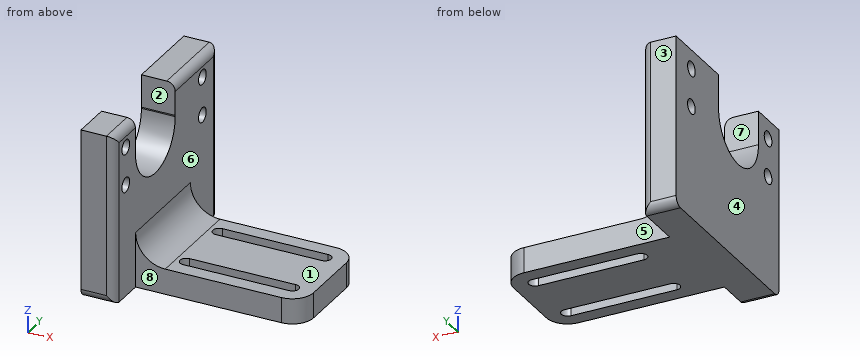
from build123d import *

# Parameters (mm, degrees)
F0_W     = 39.5
F0_H     = 25
F1_DEPTH = 6
F2_R     = 5
F3_W     = 8
F3_H     = 47
F4_DEPTH = 25
F5_R     = 7
F6_DEPTH = 40
F7_R     = 1.75
F8_DEPTH = 25
F9_R     = 2


with BuildPart() as f1:
    # F0 (on Top) → F1 (new body)
    with BuildSketch(Plane.XY):
        with Locations((19.75, -12.5)):
            Rectangle(F0_W, F0_H)
        with BuildLine():
            ThreePointArc((9.428176, -21.5), (7.928176, -20), (9.428176, -18.5))
            Line((9.428176, -18.5), (34.428176, -18.5))
            ThreePointArc((34.428176, -18.5), (36.00043, -19.963218), (34.5, -21.5))
            Line((34.5, -21.5), (9.428176, -21.5))
        make_face(mode=Mode.SUBTRACT)
        with BuildLine():
            ThreePointArc((9.428176, -6.5), (7.928176, -5), (9.428176, -3.5))
            Line((9.428176, -3.5), (34.428176, -3.5))
            ThreePointArc((34.428176, -3.5), (35.928176, -5), (34.428176, -6.5))
            Line((34.428176, -6.5), (9.428176, -6.5))
        make_face(mode=Mode.SUBTRACT)
    extrude(amount=F1_DEPTH)

    # F2
    f2_edges = [f1.edges().sort_by_distance(p)[0] for p in [
        (39.5, 0, 3),
        (39.5, -25, 3),
    ]]
    fillet(f2_edges, radius=F2_R)

    # F3 (on Top) → F4 (join)
    with BuildSketch(Plane.XY):
        with Locations((-4, -11)):
            Rectangle(F3_W, F3_H)
    extrude(amount=F4_DEPTH)

    # F5
    f5_edges = [f1.edges().sort_by_distance(p)[0] for p in [
        (0, -12.5, 6),
        (0, -34.5, 12.5),
        (0, 12.5, 12.5),
    ]]
    fillet(f5_edges, radius=F5_R)

    # F3 (on Top) → F6 (join)
    with BuildSketch(Plane.XY):
        with Locations((-4, -11)):
            Rectangle(F3_W, F3_H)
    extrude(amount=F6_DEPTH)

    # F7 (on Right) → F8 (cut)
    with BuildSketch(Plane.YZ):
        with Locations((-29.5, 35.5)):
            Circle(F7_R)
        with Locations((5.5, 35.5)):
            Circle(F7_R)
        with Locations((5.5, 26.5)):
            Circle(F7_R)
        with Locations((-29.5, 26.5)):
            Circle(F7_R)
        with BuildLine():
            ThreePointArc((-25.098021, 32), (-16, 22.901979), (-6.901979, 32))
            ThreePointArc((-6.901979, 32), (-6.903109, 32.143378), (-6.906498, 32.286721))
            ThreePointArc((-6.906498, 32.286721), (-8.276915, 36.809152), (-11.730835, 40.03419))
            Line((-11.730835, 40.03419), (-20.269165, 40.03419))
            ThreePointArc((-20.269165, 40.03419), (-23.797914, 36.686845), (-25.098021, 32))
        make_face()
        with BuildLine():
            ThreePointArc((-11.730835, 40.03419), (-8.276915, 36.809152), (-6.906498, 32.286721))
            Line((-6.906498, 32.286721), (-6.906498, 40.03419))
            Line((-6.906498, 40.03419), (-11.730835, 40.03419))
        make_face()
        with BuildLine():
            Line((-25.098021, 40.03419), (-25.098021, 32))
            ThreePointArc((-25.098021, 32), (-23.797914, 36.686845), (-20.269165, 40.03419))
            Line((-20.269165, 40.03419), (-25.098021, 40.03419))
        make_face()
        with BuildLine():
            Line((-20.269165, 40.03419), (-11.730835, 40.03419))
            ThreePointArc((-11.730835, 40.03419), (-16, 41.098021), (-20.269165, 40.03419))
        make_face()
    extrude(amount=-F8_DEPTH, mode=Mode.SUBTRACT)

    # F9
    f9_edges = [f1.edges().sort_by_distance(p)[0] for p in [
        (0, 2.796751, 40),
        (0, -29.79901, 40),
        (0, -34.5, 20),
        (0, 12.5, 20),
        (-4, 12.5, 0),
        (-4, -34.5, 0),
    ]]
    fillet(f9_edges, radius=F9_R)


solid = f1.part
Read the model definition and answer for the solid it produces. Units are mm, in the model's axes. Face numbers are marked on the shaded views. A direction names the side the tool comes from. Give positions to 0.01 mm unless a question says otherwise; leave off trailing zeros. Loops run counter-clockwise (first coordinate to the right, second up) from the corner with the lowest first, then second, coordinate; pieces in that order, holes last. Notation, with made-up numbers: (-12, 77.25) -> (-5, 77.25) arc R20 ccw to (-5, 104.25) -> close; hole circle Ø1 at (72.25, 81.5). An arc over 180 degrees is marked (long way). Use a Markdown table: item, result.
Q1. Section B-B, the plane y = 5.5 is taken. Determine the outline of the cut face in (x, z).
Solved:
| item | result |
|---|---|
| outline | (-8, 0) -> (0, 0) -> (0, 24.75) -> (-8, 24.75) -> close; (-8, 28.25) -> (0, 28.25) -> (0, 33.75) -> (-8, 33.75) -> close; (-8, 37.25) -> (0, 37.25) -> (0, 38) arc R2 ccw to (-2, 40) -> (-8, 40) -> close |
Q2. Section C-C, the plane z = 26.5 is taken. Determine the outline of the cut face in (x, y), then the cut area to 3 significant figures.
Solved:
| item | result |
|---|---|
| outline | (-8, -34.5) -> (-2, -34.5) arc R2 ccw to (0, -32.5) -> (0, -31.25) -> (-8, -31.25) -> close; (-8, -27.75) -> (0, -27.75) -> (0, -23.25) -> (-8, -23.25) -> close; (-8, -8.75) -> (0, -8.75) -> (0, 3.75) -> (-8, 3.75) -> close; (-8, 7.25) -> (0, 7.25) -> (0, 10.5) arc R2 ccw to (-2, 12.5) -> (-8, 12.5) -> close |
| area | 202 mm^2 |
Q3. Determine the mould class of the marked faces 6, 7 and 8 for opening direction Y: pulls with the +Y half, pulls with the -Y half, needs draft (parallel to the pull), parting line crosses it, or undercut.
Solved:
| item | result |
|---|---|
| face 6 | needs draft |
| face 7 | undercut |
| face 8 | pulls with the -Y half |
Q4. Section A-A, the plane x = 12 is taken. Determine the outline of the cut face in (y, z), then the cut area to 3 significant figures.
Solved:
| item | result |
|---|---|
| outline | (-25, 0) -> (-21.5, 0) -> (-21.5, 6) -> (-25, 6) -> close; (-18.5, 0) -> (-6.5, 0) -> (-6.5, 6) -> (-18.5, 6) -> close; (-3.5, 0) -> (0, 0) -> (0, 6) -> (-3.5, 6) -> close |
| area | 114 mm^2 |
Q5. Each of these flat-tipped pins is pushed along its axis until it touches: pin 1 (4 mm diameter, centred on x = 10, z = 8.5, fed in from +Y); pin 2 (1.5 mm diameter, centred on x = 13.5, y = -8, fed in from +Z); pin 3 (12 mm diameter, centred on y = -5, z = 32, fed in from +X); pin 4 (1.8 mm diameter, centred on x = 27, z = 3, fed in from +Y). Where does it stop, or does it pass through?
Solved:
| item | result |
|---|---|
| pin 1 | passes through |
| pin 2 | stops at z = 6 |
| pin 3 | stops at x = 0 |
| pin 4 | stops at y = 0 |
Q6. A tool of negligible diameter and unlimited length cuts with its end or side. For the marked faces 1, 2, 3, 4 and 5, from which of +Z, -Z, +X, -X, +Y, -Y can it reach the whole face along a straight path? Write none if from no direction.
Solved:
| item | result |
|---|---|
| face 1 | +Z, +X, +Y, -Y |
| face 2 | +Z, +X, -X |
| face 3 | +Z, -Z, +X, -X, +Y |
| face 4 | +Z, -Z, -X, +Y, -Y |
| face 5 | +Z, -Z, +X, +Y |
Q7. Section D-D, the plane y = -16 is taken. Determine the outline of the cut face in (x, z), then the cut area to 3 significant figures.
Solved:
| item | result |
|---|---|
| outline | (-8, 0) -> (39.5, 0) -> (39.5, 6) -> (7, 6) arc R7 cw to (0, 13) -> (0, 22.9) -> (-8, 22.9) -> close |
| area | 431 mm^2 |
Q8. Find the intervals of material crossed by line 1 along Z through (x, y) = (-4, -29.5); line 2 along Y through (x, z) = (-4, 26); line 3 along Z through (x, y) = (32, -9), in increasing order.
Solved:
| item | result |
|---|---|
| line 1 | z = 0 to 24.75, 28.25 to 33.75, 37.25 to 40 |
| line 2 | y = -34.5 to -31.18, -27.82 to -22.84, -9.16 to 3.82, 7.18 to 12.5 |
| line 3 | z = 0 to 6 |
